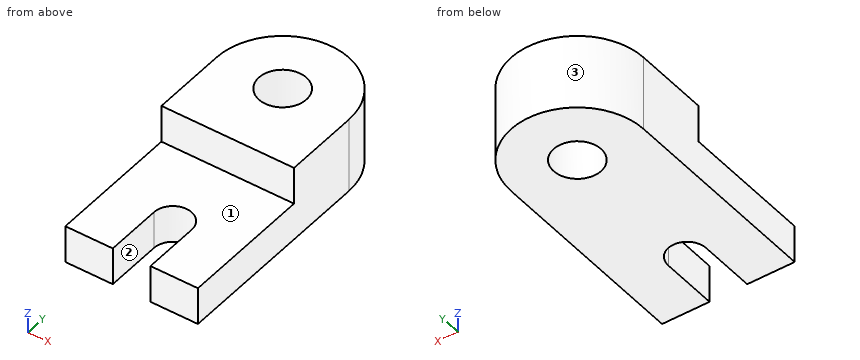
```python
from build123d import *

# Parameters (mm, degrees)
F1_DEPTH = 12.7
F3_DEPTH = 12.7
F5_D     = 16.002


with BuildPart() as f1:
    # F0 (on Top) → F1 (new body)
    with BuildSketch(Plane.XY):
        with BuildLine():
            Line((-5.128147, -40.08238), (-5.128147, 29.76762))
            ThreePointArc((-5.128147, 29.76762), (-27.480147, 52.11962), (-49.832147, 29.76762))
            Line((-49.832147, 29.76762), (-49.832147, -40.08238))
            Line((-49.832147, -40.08238), (-33.830147, -40.08238))
            Line((-33.830147, -40.08238), (-33.830147, -21.03238))
            ThreePointArc((-33.830147, -21.03238), (-27.480147, -14.68238), (-21.130147, -21.03238))
            Line((-21.130147, -21.03238), (-21.130147, -40.08238))
            Line((-21.130147, -40.08238), (-5.128147, -40.08238))
        make_face()
    extrude(amount=F1_DEPTH)

    # F2 (on face) → F3 (join)
    with BuildSketch(Plane.XY.offset(12.7)):
        with BuildLine():
            Line((-49.832147, 29.76762), (-49.832147, 4.36762))
            Line((-49.832147, 4.36762), (-5.128147, 4.36762))
            Line((-5.128147, 4.36762), (-5.128147, 29.76762))
            ThreePointArc((-5.128147, 29.76762), (-27.480147, 52.11962), (-49.832147, 29.76762))
        make_face()
    extrude(amount=F3_DEPTH)

    # F5 (through all)
    with Locations(Plane.XY.offset(25.4)):
        with Locations((-27.480147, 29.76762)):
            Hole(F5_D / 2)


solid = f1.part
```
Check sheet for the modelled part. Datum: model origin and axes. Units: mm. Face numbers are marked on the shaded views. A direction names the side the tool comes from. Round coordinates to 2 decimals unless told otherwise and drop trailing zeros. Order: outer loops, then holes, each group sorted by start corner. A loop starts at its lowest first (then second) coordinate and runs counter-clockwise, first axis right, second up.
1) Section check A-A (y = -31.5). Record the boundary of the cut face in (x, z), and give its area (3 significant figures).
2) Go/stop test with flat-tipped pins: pin 1 Ø5 at (x, z) = (-12, 18.5) entering from -Y; pin 2 Ø1 at (x, z) = (-14, 4) entering from +Y; pin 3 Ø22 at (x, y) = (-33, -14.5) entering from +Z. Record where each tip stops, or that it passes through.
3) Section check B-B (z = 2.5). Record the boundary of the cut face in (x, y).
4) Scan lines: line 1 (X direction, y = -27.5, z = 1.5); line 2 (Z direction, x = -19.5, y = 4); line 3 (Y direction, x = -24.5, z = 22.5). Record each from-to range of solid material in increasing order.
5) Tool access check on the marked faces 1, 2 and 3. Record the directions out of +Z, -Z, +X, -X, +Y, -Y that give a thin tool (end or side, any length) a straight path to the whole face; none if there is none.
6) Section check D-D (y = 33). Record the boundary of the cut face in (x, z), and give its area (3 significant figures).
7) Section check C-C (x = -24). Record the boundary of the cut face in (y, z), and give its area (3 significant figures).
Result:
1. outline: (-49.83, 0) - (-33.83, 0) - (-33.83, 12.7) - (-49.83, 12.7) - close; (-21.13, 0) - (-5.13, 0) - (-5.13, 12.7) - (-21.13, 12.7) - close
1. area: 406 mm2
2. pin 1: stops at y = 4.37
2. pin 2: stops at y = 47.96
2. pin 3: stops at z = 12.7
3. outline: (-49.83, -40.08) - (-33.83, -40.08) - (-33.83, -21.03) arc R6.35 cw to (-21.13, -21.03) - (-21.13, -40.08) - (-5.13, -40.08) - (-5.13, 29.77) arc R22.35 ccw to (-49.83, 29.77) - close; hole circle Ø16 at (-27.48, 29.77)
4. line 1: x = -49.83 to -33.83, -21.13 to -5.13
4. line 2: z = 0 to 12.7
4. line 3: y = 4.37 to 22.34, 37.19 to 51.92
5. face 1: +Z, +X, -X, -Y
5. face 2: +Z, -Z, -Y
5. face 3: +Z, -Z, +Y
6. outline: (-49.6, 0) - (-34.8, 0) - (-34.8, 25.4) - (-49.6, 25.4) - close; (-20.16, 0) - (-5.36, 0) - (-5.36, 25.4) - (-20.16, 25.4) - close
6. area: 752 mm2
7. outline: (-15.72, 0) - (22.56, 0) - (22.56, 25.4) - (4.37, 25.4) - (4.37, 12.7) - (-15.72, 12.7) - close; (36.97, 0) - (51.85, 0) - (51.85, 25.4) - (36.97, 25.4) - close
7. area: 1,100 mm2
